The listing builds one solid part. Answer for the finished solid, in the listing's coordinates (mm). A direction names the side the tool comes from. Coordinates: 2 decimals unless noted, no trailing zeros. Loops run counter-clockwise (first coordinate to the right, second up) from the corner with the lowest first, then second, coordinate; pieces in that order, holes last. Notation, with made-up numbers: (76.25, 48.25) - (132.25, 48.25) arc R12 ccw to (132.25, 63.25) - close; hole circle Ø5 at (7, 23). An arc over 180 degrees is marked (long way). Use one line per item in the form item = value. Start each with the question number.
Autodesk Fusion 360 part; units mm, degrees
sketch "Sketch1" plane through (0, 0, 0) normal (0, 0, 1) x (1, 0, 0)
  circle A0 centre (0, 0) radius 3
  circle A1 centre (0, 0) radius 1.25
  circle A2 centre (0, 0) radius 7.5
  circle A3 centre (-7.5, 0.0183) radius 6.93
  circle A4 centre (-7.5, 0.0183) radius 4.9285
  dimension "d1" = 6
  dimension "d2" = 2.5
  dimension "d3" = 15
extrude "Extrude1" add sketch "Sketch1" along normal blind 10 contours A0 A1 A3 | A0 A1 A3 A4 | A0 A4
extrude "Extrude2" add sketch "Sketch1" along normal blind 3 contours A0 A2 A3 | A0 A2 A3 A4 | A0 A2 A3 A4 | A0 A2 A4 | A1 A3 | A1 A3
fillet "Fillet1" radius 1.25 1 edges at (-2.797, -1.0848, 10)
extrude "Extrude3" add sketch "Sketch1" along normal blind 3 contours A2 A3 A4
fillet "Fillet2" radius 1 2 edges at (-5.892, -4.6405, 1.5) (-5.8693, 4.6692, 1.5)
fillet "Fillet3" radius 1 4 edges at (-6.6744, 4.4673, 3) (-12.4284, 0.0303, 3) (-6.6961, -4.4347, 3) (-7.5, 0.0183, 3)
fillet "Fillet4" radius 1 1 edges at (-14.43, 0.0352, 3)
(1) For faces 1 (the face through (-7.5, 0, 1)), 2 (the face through (-3, 0, 6)), 3 (the face through (-4, 0, 0)), determine the directions among +Z, -Z, +X, -X, +Y, -Y from which every point of the face is accessible in a straight line to the end or side of a thin tool.
(2) A cutting plane is placed at A-A (x = 0). Determine the outline of the cut face in (y, z).
(3) Determine the mould class of faces 4 (the face through (0, 0, 3)), 5 (the face through (7.497, 0.226, 1.479)), 6 (the face through (-1, 3, 3)) for opening direction Y: +Y half, -Y half, draft (parallel to the pull), parting line (faces both ways), or undercut.
(4) A cutting plane is placed at B-B (z = 5.5). Determine the outline of the cut face in (x, y), then the cut area to 3 significant figures.
(5) A cutting plane is placed at C-C (z = 9.25). Determine the outline of the cut face in (x, y).
(6) Find the intervals of material crossed by probe 1 along X at (y, z) = (0, 4.5); probe 2 along Z at (x, y) = (5, -1); probe 3 along X at (y, z) = (-1, 5.25), in increasing order. Write a range as from..to.
(7) Each of these flat-tipped pins is pushed along its axis until it touches: pin 1 Ø6 at (y, z) = (2, 7.5) entering from -X; pin 2 Ø6 at (x, y) = (-3.5, -4.5) entering from +Z; pin 3 Ø1.2 at (x, y) = (-0.5, 0) entering from +Z. Where does it stop, or does it pass through?
Evaluation:
q1.face_1 = +Z, -Z
q1.face_2 = +Z
q1.face_3 = -Z, +X, -X, +Y, -Y
q2.outline = (-7.5, 0) - (7.5, 0) - (7.5, 3) - (3, 3) - (3, 8.75) arc R1.25 ccw to (1.75, 10) - (1.25, 10) - (1.25, 3) - (-1.25, 3) - (-1.25, 10) - (-1.75, 10) arc R1.25 ccw to (-3, 8.75) - (-3, 3) - (-7.5, 3) - close
q3.face_4 = undercut
q3.face_5 = parting line
q3.face_6 = draft
q4.outline = circle Ø6 at (0, 0); hole circle Ø2.5 at (0, 0)
q4.area = 23.4 mm^2
q5.outline = circle Ø5.79 at (0, 0); hole circle Ø2.5 at (0, 0)
q6.probe_1 = -3..-1.25, 1.25..3
q6.probe_2 = 0..3
q6.probe_3 = -2.83..-0.75, 0.75..2.83
q7.pin_1 = -3
q7.pin_2 = 9.56
q7.pin_3 = 3
